Autodesk Inventor part; units mm, degrees
ref_plane "YZ Plane" through (0, 0, 0) normal (1, 0, 0) x (0, 1, 0)
ref_plane "XZ Plane" through (0, 0, 0) normal (0, 1, 0) x (-1, 0, 0)
ref_plane "XY Plane" through (0, 0, 0) normal (0, 0, 1) x (1, 0, 0)
sketch "Sketch1" plane through (0, 0, 0) normal (0, 0, 1) x (1, 0, 0)
  line L0 (-42.0848, 28.5) -> (-42.0848, 31.5)
  line L1 (-24.5848, 28.5) -> (-42.0848, 28.5)
  line L2 (-24.5848, 31.5) -> (-24.5848, 28.5)
  line L3 (-24.5848, 31.5) -> (24.5848, 31.5)
  line L4 (24.5848, 28.5) -> (24.5848, 31.5)
  line L5 (42.0848, 28.5) -> (24.5848, 28.5)
  line L6 (42.0848, 31.5) -> (42.0848, 28.5)
  circle A0 centre (-45.2648, 16.1838) radius 8.115
  circle A1 centre (-22.4048, 16.1838) radius 8.115
  circle A2 centre (-14.7848, 23.4228) radius 1.5875
  circle A3 centre (-52.8848, 8.9448) radius 1.5875
  circle A4 centre (-33.8348, 9.5798) radius 2.5
  circle A5 centre (14.7848, 8.9448) radius 1.5875
  circle A6 centre (22.4048, 16.1838) radius 8.115
  circle A7 centre (33.8348, 9.5798) radius 2.5
  circle A8 centre (45.2648, 16.1838) radius 8.115
  circle A9 centre (52.8848, 23.4228) radius 1.5875
  line L7 (-60.406, 31.5) -> (60.406, -31.5) construction
  line L8 (60.406, 31.5) -> (-60.406, -31.5) construction
  line L9 (-7.5, -31.5) -> (7.5, -31.5)
  line L10 (7.5, -31.5) -> (7.5, -28.5)
  line L11 (-7.5, -28.5) -> (-7.5, -31.5)
  line L12 (-7.5, -31.5) -> (7.5, -28.5) construction
  line L13 (7.5, -31.5) -> (-7.5, -28.5) construction
  line L14 (0, 0) -> (13.8, 0) construction
  line L15 (13.8, 0) -> (13.8, 4) construction
  line L16 (-30.5, -31.5) -> (-15.5, -31.5)
  line L17 (-53.5, -31.5) -> (-38.5, -31.5)
  line L18 (15.5, -31.5) -> (30.5, -31.5)
  line L19 (-7.5, -31.5) -> (7.5, -31.5)
  line L20 (-30.5, -31.5) -> (-15.5, -31.5)
  line L21 (38.5, -31.5) -> (53.5, -31.5)
  line L22 (15.5, -31.5) -> (30.5, -31.5)
  line L23 (-7.5, -31.5) -> (7.5, -31.5)
  line L24 (-15.5, -31.5) -> (-15.5, -28.5)
  line L25 (-15.5, -28.5) -> (-7.5, -28.5)
  line L26 (-30.5, -31.5) -> (-30.5, -28.5)
  line L27 (-30.5, -28.5) -> (-38.5, -28.5)
  line L28 (-38.5, -28.5) -> (-38.5, -31.5)
  line L29 (-53.5, -31.5) -> (-53.5, -28.5)
  line L30 (15.5, -31.5) -> (15.5, -28.5)
  line L31 (15.5, -28.5) -> (7.5, -28.5)
  line L32 (30.5, -31.5) -> (30.5, -28.5)
  line L33 (30.5, -28.5) -> (38.5, -28.5)
  line L34 (38.5, -31.5) -> (38.5, -28.5)
  line L35 (53.5, -31.5) -> (53.5, -28.5)
  line L36 (-60.4057, -31.5) -> (-60.4057, -31.4998)
  line L37 (-63.4057, 5) -> (-63.4057, 15)
  line L38 (-63.4057, -5) -> (-63.4057, -15)
  line L39 (-63.4057, -25) -> (-63.4057, -28.5)
  line L40 (-63.4057, 25) -> (-63.4057, 31.5)
  line L41 (-42.0848, 31.5) -> (-63.4057, 31.5)
  line L42 (-63.4057, 25) -> (-60.4057, 25)
  line L43 (-60.4057, 25) -> (-60.4057, 15)
  line L44 (-63.4057, 15) -> (-60.4057, 15)
  line L45 (-63.4057, 5) -> (-60.4057, 5)
  line L46 (-60.4057, 5) -> (-60.4057, -5)
  line L47 (-60.4057, -5) -> (-63.4057, -5)
  line L48 (-63.4057, -15) -> (-60.4057, -15)
  line L49 (-60.4057, -15) -> (-60.4057, -25)
  line L50 (-60.4057, -25) -> (-63.4057, -25)
  line L51 (-63.4057, -28.5) -> (-53.5, -28.5)
  line L52 (0, 0) -> (0, 18) construction
  line L53 (60.4057, -31.5) -> (60.4057, -31.4998)
  line L54 (63.4057, 5) -> (63.4057, 15)
  line L55 (63.4057, -5) -> (63.4057, -15)
  line L56 (63.4057, -25) -> (63.4057, -28.5)
  line L57 (63.4057, 25) -> (63.4057, 31.5)
  line L58 (42.0848, 31.5) -> (63.4057, 31.5)
  line L59 (63.4057, 25) -> (60.4057, 25)
  line L60 (60.4057, 25) -> (60.4057, 15)
  line L61 (63.4057, 15) -> (60.4057, 15)
  line L62 (63.4057, 5) -> (60.4057, 5)
  line L63 (60.4057, 5) -> (60.4057, -5)
  line L64 (60.4057, -5) -> (63.4057, -5)
  line L65 (63.4057, -15) -> (60.4057, -15)
  line L66 (60.4057, -15) -> (60.4057, -25)
  line L67 (60.4057, -25) -> (63.4057, -25)
  line L68 (63.4057, -28.5) -> (53.5, -28.5)
  point P0 (0, 0)
  point P1 (0, -30)
  dimension "d0" = 15
  dimension "d1" = 3
  dimension "d5" = 23
  dimension "d8" = 23
  dimension "d11" = 3
  dimension "d12" = 3
  dimension "d13" = 90
  dimension "d14" = 3
  dimension "d17" = 3
  dimension "d18" = 10
  dimension "d20" = 10
extrude "Extrusion1" add sketch "Sketch1" along normal mid plane 3
properties part number "srfbelakang"
CAD build for the part. Positions are in the model's coordinates, mm. A direction names the side the tool comes from. Round coordinates to 2 decimals unless told otherwise and drop trailing zeros. Loops run counter-clockwise (first coordinate to the right, second up) from the corner with the lowest first, then second, coordinate; pieces in that order, holes last.
(1) Two-plate mould, pull along Y, no slides. Class faces 5 (the flat face through (-53, 31.5, 0)), 6 (the flat face through (46, -31.5, 0)), 7 (the flat face through (-62, -5, 0)), 8 (the flat face through (60.406, 20, 0)): +Y half, -Y half, draft (parallel to the pull), parting line (faces both ways), or undercut.
(2) Cut at B-B (y = 19). Give the cut face in (x, z).
(3) Cut at D-D (z = -0.4). State how many separate pieces and enclosed holes the cut face has, plus the area to 3 significant figures.
(4) Cut at A-A (x = -33). Give the cut face in (y, z), plus the area to 3 significant figures.
(5) Wall check: line 1 along Y through (x, z) = (-45, -1.05); line 2 along X through (y, z) = (14, -0.3); line 3 along X through (y, z) = (-15.5, 0.2). Give the ranges that are in metal, low to high.
(6) Cut at C-C (x = 9). Give the cut face in (y, z).
(7) Which spindle directions (+Z, -Z, +X, -X, +Y, -Y) get a long thin tool onto all of the face, cutting with end or side? Do faces 1 (the flat face through (-33, 28.5, 0)), 2 (the flat face through (-62, 5, 0)), 3 (the flat face through (-12, -28.5, 0)), 4 (the flat face through (60.406, -20, 0)). Say none if no direction does.
(8) Drop flat-ended pins along their axis: pin 1 (1.5 mm diameter, centred on y = 19.5, z = -0.5, fed in from -X); pin 2 (21 mm diameter, centred on x = 22.4, y = 16.18, fed in from -Z); pin 3 (0.9 mm diameter, centred on x = -57, z = -0.5, fed in from -Y); pin 4 (1.5 mm diameter, centred on y = -30.5, z = 0, fed in from -X). Give the stop position or say it passes through.
Findings below:
1. face 5: +Y half
1. face 6: -Y half
1. face 7: undercut
1. face 8: undercut
2. outline: (-60.41, -1.5) - (-52.88, -1.5) - (-52.88, 1.5) - (-60.41, 1.5) - close; (-37.65, -1.5) - (-30.02, -1.5) - (-30.02, 1.5) - (-37.65, 1.5) - close; (-14.79, -1.5) - (14.79, -1.5) - (14.79, 1.5) - (-14.79, 1.5) - close; (30.02, -1.5) - (37.65, -1.5) - (37.65, 1.5) - (30.02, 1.5) - close; (52.88, -1.5) - (60.41, -1.5) - (60.41, 1.5) - (52.88, 1.5) - close
3. separate pieces: 1
3. enclosed holes: 10
3. area: 6,650 mm2
4. outline: (-28.5, -1.5) - (7.22, -1.5) - (7.22, 1.5) - (-28.5, 1.5) - close; (11.94, -1.5) - (28.5, -1.5) - (28.5, 1.5) - (11.94, 1.5) - close
4. area: 157 mm2
5. line 1: y = -31.5 to 8.07, 24.29 to 31.5
5. line 2: x = -63.41 to -53.08, -37.45 to -30.22, -14.59 to 14.59, 30.22 to 37.45, 53.08 to 63.41
5. line 3: x = -60.41 to 60.41
6. outline: (-28.5, -1.5) - (31.5, -1.5) - (31.5, 1.5) - (-28.5, 1.5) - close
7. face 1: +Z, -Z, +Y
7. face 2: +Z, -Z, -X
7. face 3: +Z, -Z, -Y
7. face 4: +Z, -Z, +X
8. pin 1: stops at x = -60.41
8. pin 2: stops at z = -1.5
8. pin 3: stops at y = -28.5
8. pin 4: stops at x = -53.5
